Here's how the part is built. I have some questions about the finished solid (model axes, mm). A direction names the side the tool comes from. Give positions to 0.01 mm unless a question says otherwise; leave off trailing zeros. Loops run counter-clockwise (first coordinate to the right, second up) from the corner with the lowest first, then second, coordinate; pieces in that order, holes last.
Q1. If we section it at B-B (x = 137.5): Please give me the cut outline in (y, z), plus the area to 3 significant figures.
Q2. I need wall thicknesses on line 1 (Z direction, x = 55.5, y = 79); line 2 (Z direction, x = 125, y = -4). Which ranges of each line are inside material? Lowest first, please.
Q3. Will these pins go through, and if not, where does the flat tip stop? P1, Ø12, axis at x = 158, y = 24.5, coming from the +Z side; P2, Ø2, axis at y = 20, z = -67, coming from the -X side.
Q4. If we section it at C-C (y = 6): Please give me the cut outline in (x, z), plus the area to 3 significant figures.
Q5. If we section it at D-D (x = 51): Please give me the cut outline in (y, z).
Q6. For faces 1 (the face through (120.99, 76.27, -65.03)), 2 (the face through (89, 80.004, -57)), 3 (the face through (71.7, 42.61, -51.82)), which set-ups out of +Z, -Z, +X, -X, +Y, -Y let a thin tool reach every point of the face, with its end or its side?
Q7. If we section it at A-A (x = 114): Please give me the cut outline in (y, z), plus the area to 3 significant figures.
Q8. We'd pull the mould along X, two halves only. Please class faces 4 (the face through (105.77, 45.77, -59.38)), 5 (the face through (121.688, 0.097, -65.219)), 6 (the face through (105, -9.996, -61)): +X half, -X half, draft (parallel to the pull), parting line (faces both ways), or undercut.
from build123d import *

# Parameters (mm, degrees)
SKETCH2_W      = 140
SKETCH2_H      = 110
SKETCH2_R      = 1.6
SKETCH2_R_2    = 2.1
EXTRUDE1_DEPTH = 3


with BuildPart() as part:
    # Sketch2 → Extrude1 (new body)
    with BuildSketch(Plane(origin=(-8.535929163, 0, -31.856521324), x_dir=(0.9659258262890755, 0, -0.2588190451024938), z_dir=(0.2588190451024938, 0, 0.9659258262890756))):
        with Locations((118.519484346, 45.004395502)):
            Rectangle(SKETCH2_W, SKETCH2_H)
        with Locations((166.519484346, 92.504395502)):
            Circle(SKETCH2_R, mode=Mode.SUBTRACT)
        with Locations((146.519484346, 92.504395502)):
            Circle(SKETCH2_R, mode=Mode.SUBTRACT)
        with Locations((146.519484346, -2.495604498)):
            Circle(SKETCH2_R, mode=Mode.SUBTRACT)
        with Locations((166.519484346, -2.495604498)):
            Circle(SKETCH2_R, mode=Mode.SUBTRACT)
        with Locations((176.519484346, 0.004395502)):
            Circle(SKETCH2_R_2, mode=Mode.SUBTRACT)
        with Locations((136.519484346, 0.004395502)):
            Circle(SKETCH2_R_2, mode=Mode.SUBTRACT)
        with Locations((176.519484346, 90.004395502)):
            Circle(SKETCH2_R_2, mode=Mode.SUBTRACT)
        with Locations((136.519484346, 90.004395502)):
            Circle(SKETCH2_R_2, mode=Mode.SUBTRACT)
        with BuildLine():
            Line((71.422427124, 72.331747658), (94.235598815, 12.035198256))
            ThreePointArc((94.235598815, 12.035198256), (94.06679625, 10.651812407), (92.832656037, 10.004395502))
            Line((92.832656037, 10.004395502), (70.019484346, 10.004395502))
            ThreePointArc((70.019484346, 10.004395502), (68.958824174, 10.44373533), (68.519484346, 11.504395502))
            Line((68.519484346, 11.504395502), (68.519484346, 71.800944904))
            ThreePointArc((68.519484346, 71.800944904), (69.749682721, 73.276481106), (71.422427124, 72.331747658))
        make_face(mode=Mode.SUBTRACT)
        with BuildLine():
            Line((81.382592108, 80.004395502), (121.278221323, 80.004395502))
            ThreePointArc((121.278221323, 80.004395502), (122.460552573, 79.427484239), (122.73341687, 78.140519257))
            Line((122.73341687, 78.140519257), (106.858201548, 14.653157981))
            ThreePointArc((106.858201548, 14.653157981), (105.490462864, 13.519585964), (104.000063225, 14.486231472))
            Line((104.000063225, 14.486231472), (79.979649331, 77.973592748))
            ThreePointArc((79.979649331, 77.973592748), (80.148451895, 79.356978598), (81.382592108, 80.004395502))
        make_face(mode=Mode.SUBTRACT)
        with BuildLine():
            Line((168.519484346, 78.504395502), (168.519484346, 18.857688255))
            ThreePointArc((168.519484346, 18.857688255), (167.270056066, 17.378765061), (165.603199262, 18.363586484))
            Line((165.603199262, 18.363586484), (144.794151706, 78.010293731))
            ThreePointArc((144.794151706, 78.010293731), (144.987499209, 79.372971159), (146.210436791, 80.004395502))
            Line((146.210436791, 80.004395502), (167.019484346, 80.004395502))
            ThreePointArc((167.019484346, 80.004395502), (168.080144518, 79.565055674), (168.519484346, 78.504395502))
        make_face(mode=Mode.SUBTRACT)
        with BuildLine():
            Line((132.289557089, 75.134147375), (116.469724954, 11.868271747))
            ThreePointArc((116.469724954, 11.868271747), (116.742589251, 10.581306765), (117.924920501, 10.004395502))
            Line((117.924920501, 10.004395502), (155.81642558, 10.004395502))
            ThreePointArc((155.81642558, 10.004395502), (157.039363161, 10.635819845), (157.232710664, 11.998497273))
            Line((157.232710664, 11.998497273), (135.16103772, 75.2643729))
            ThreePointArc((135.16103772, 75.2643729), (133.676795459, 76.268730946), (132.289557089, 75.134147375))
        make_face(mode=Mode.SUBTRACT)
        with BuildLine():
            ThreePointArc((54.043190493, -2.495604498), (55.693190493, -4.145604498), (57.343190493, -2.495604498))
            ThreePointArc((57.343190493, -2.495604498), (55.693190493, -0.845604498), (54.043190493, -2.495604498))
        make_face(mode=Mode.SUBTRACT)
        with BuildLine():
            ThreePointArc((79.043190493, -2.495604498), (80.693190493, -4.145604498), (82.343190493, -2.495604498))
            ThreePointArc((82.343190493, -2.495604498), (80.693190493, -0.845604498), (79.043190493, -2.495604498))
        make_face(mode=Mode.SUBTRACT)
        with BuildLine():
            ThreePointArc((79.043190493, 92.504395502), (80.693190493, 90.854395502), (82.343190493, 92.504395502))
            ThreePointArc((82.343190493, 92.504395502), (80.693190493, 94.154395502), (79.043190493, 92.504395502))
        make_face(mode=Mode.SUBTRACT)
        with BuildLine():
            ThreePointArc((54.043190493, 92.504395502), (55.693190493, 90.854395502), (57.343190493, 92.504395502))
            ThreePointArc((57.343190493, 92.504395502), (55.693190493, 94.154395502), (54.043190493, 92.504395502))
        make_face(mode=Mode.SUBTRACT)
    extrude(amount=EXTRUDE1_DEPTH)


solid = part.part
Check sheet entries:
1. outline: (-10, -70.99) - (10, -70.99) - (10, -67.88) - (-10, -67.88) - close; (29.33, -70.99) - (59.68, -70.99) - (61.99, -67.88) - (31.63, -67.88) - close; (80, -70.99) - (100, -70.99) - (100, -67.88) - (80, -67.88) - close
1. area: 219 mm2
2. line 1: z = -49.01 to -45.91
2. line 2: z = -67.64 to -64.53
3. P1: stops at z = -72.57
3. P2: passes through
4. outline: (38.33, -44.41) - (173.56, -80.65) - (174.34, -77.75) - (39.11, -41.52) - close
4. area: 420 mm2
5. outline: (-10, -47.81) - (100, -47.81) - (100, -44.7) - (-10, -44.7) - close
6. face 1: none
6. face 2: +Z, -Z
6. face 3: +Z
7. outline: (-10, -64.69) - (10, -64.69) - (10, -61.58) - (-10, -61.58) - close; (50.2, -61.58) - (53.41, -64.69) - (100, -64.69) - (100, -61.58) - close
7. area: 212 mm2
8. face 4: +X half
8. face 5: undercut
8. face 6: draft
